Design review of the part built by this model. Coordinates are the model's own, in mm. Coordinates: 2 decimals unless noted, no trailing zeros. Loops run counter-clockwise (first coordinate to the right, second up) from the corner with the lowest first, then second, coordinate; pieces in that order, holes last. Notation, with made-up numbers: M 16.25,-12.75 L 53.25,-12.75 A10 ccw 53.25,-4.75 Z; hole C 20,37.25 d9. An arc over 180 degrees is marked long. Answer as CSV lines item,"result". Start each with the question number.
from build123d import *

# Parameters (mm, degrees)
SKETCH_1_R             = 175
EXTRUDE_1_DEPTH        = 3
CUT_EXTRUDE_1_DEPTH    = 3
FILLET_1_R             = 5
FILLET_2_R             = 5
FILLET_3_R             = 5
SKETCH_5_R             = 1.5
CUT_EXTRUDE_4_DEPTH    = 3
SKETCH_6_R             = 1.5
CUT_EXTRUDE_5_DEPTH    = 3
SKETCH_7_W             = 30
SKETCH_7_H             = 108
CUT_EXTRUDE_6_DEPTH    = 3
SKETCH_8_R             = 1.5
CUT_EXTRUDE_7_DEPTH    = 3
SKETCH_9_R             = 1.5
CUT_EXTRUDE_8_DEPTH    = 10
SKETCH_10_R            = 1.6
CUT_EXTRUDE_9_DEPTH    = 10
SKETCH_11_W            = 15
SKETCH_11_H            = 30
CUT_EXTRUDE_10_DEPTH   = 10
SKETCH_17_R            = 1.5
CUT_EXTRUDE_12_DEPTH   = 4
SKETCH_29_R            = 1.5
CUT_EXTRUDE_6879_DEPTH = 4
SKETCH_30_R            = 1.5
CUT_EXTRUDE_7056_DEPTH = 4
SKETCH_31_R            = 1.5
CUT_EXTRUDE_7256_DEPTH = 4
SKETCH_32_R            = 1.5
WEB_DEPTH              = 4


with BuildPart() as part:
    # ｽｹｯﾁ1 → ﾎﾞｽ - 押し出し1 (new body)
    with BuildSketch(Plane.XY):
        Circle(SKETCH_1_R)
    extrude(amount=EXTRUDE_1_DEPTH)

    # ｽｹｯﾁ2 → ｶｯﾄ - 押し出し1 (cut)
    with BuildSketch(Plane.XY.offset(3)):
        with BuildLine():
            Line((-60, 115), (0, 115))
            Line((0, 115), (0, 175))
            ThreePointArc((0, 175), (-30.465194158, 172.327803749), (-60, 164.392822228))
            Line((-60, 164.392822228), (-60, 115))
        make_face()
        with BuildLine():
            Line((0, 175), (0, 115))
            Line((0, 115), (60, 115))
            Line((60, 115), (60, 164.392822228))
            ThreePointArc((60, 164.392822228), (30.465194158, 172.327803749), (0, 175))
        make_face()
        with BuildLine():
            Line((0, -175), (0, -115))
            Line((0, -115), (-60, -115))
            Line((-60, -115), (-60, -164.392822228))
            ThreePointArc((-60, -164.392822228), (-30.465194158, -172.327803749), (0, -175))
        make_face()
        with BuildLine():
            Line((60, -115), (0, -115))
            Line((0, -115), (0, -175))
            ThreePointArc((0, -175), (30.465194158, -172.327803749), (60, -164.392822228))
            Line((60, -164.392822228), (60, -115))
        make_face()
    extrude(amount=-CUT_EXTRUDE_1_DEPTH, mode=Mode.SUBTRACT)

    # ﾌｨﾚｯﾄ1
    fillet_1_edges = [part.edges().sort_by_distance(p)[0] for p in [
        (-60, 164.392822228, 1.5),
    ]]
    fillet(fillet_1_edges, radius=FILLET_1_R)

    # ﾌｨﾚｯﾄ2
    fillet_2_edges = [part.edges().sort_by_distance(p)[0] for p in [
        (-60, 115, 1.5),
        (60, 164.392822228, 1.5),
        (60, 115, 1.5),
    ]]
    fillet(fillet_2_edges, radius=FILLET_2_R)

    # ﾌｨﾚｯﾄ3
    fillet_3_edges = [part.edges().sort_by_distance(p)[0] for p in [
        (-60, -115, 1.5),
        (60, -115, 1.5),
        (60, -164.392822228, 1.5),
        (-60, -164.392822228, 1.5),
    ]]
    fillet(fillet_3_edges, radius=FILLET_3_R)

    # ｽｹｯﾁ5 → ｶｯﾄ - 押し出し4 (cut)
    with BuildSketch(Plane.XY.offset(3)):
        with Locations((-100, -115)):
            Circle(SKETCH_5_R)
        with Locations((100, -115)):
            Circle(SKETCH_5_R)
        with Locations((100, 115)):
            Circle(SKETCH_5_R)
        with Locations((-100, 115)):
            Circle(SKETCH_5_R)
    extrude(amount=-CUT_EXTRUDE_4_DEPTH, mode=Mode.SUBTRACT)

    # ｽｹｯﾁ6 → ｶｯﾄ - 押し出し5 (cut)
    with BuildSketch(Plane.XY.offset(3)):
        with Locations((-60, 54)):
            Circle(SKETCH_6_R)
        with Locations((60, 54)):
            Circle(SKETCH_6_R)
        with Locations((-60, -54)):
            Circle(SKETCH_6_R)
        with Locations((60, -54)):
            Circle(SKETCH_6_R)
    extrude(amount=-CUT_EXTRUDE_5_DEPTH, mode=Mode.SUBTRACT)

    # ｽｹｯﾁ7 → ｶｯﾄ - 押し出し6 (cut)
    with BuildSketch(Plane.XY.offset(3)):
        with Locations((-85, 0)):
            Rectangle(SKETCH_7_W, SKETCH_7_H)
    extrude(amount=-CUT_EXTRUDE_6_DEPTH, mode=Mode.SUBTRACT)

    # ｽｹｯﾁ8 → ｶｯﾄ - 押し出し7 (cut)
    with BuildSketch(Plane.XY.offset(3)):
        with Locations((-115, -67)):
            Circle(SKETCH_8_R)
        with Locations((-116.822468618, 0)):
            Circle(SKETCH_8_R)
        with Locations((-115, 67)):
            Circle(SKETCH_8_R)
    extrude(amount=-CUT_EXTRUDE_7_DEPTH, mode=Mode.SUBTRACT)

    # ｽｹｯﾁ9 → ｶｯﾄ - 押し出し8 (cut)
    with BuildSketch(Plane.XY.offset(3)):
        with Locations((-65, 37)):
            Circle(SKETCH_9_R)
        with Locations((20, 41)):
            Circle(SKETCH_9_R)
        with Locations((-65, -38)):
            Circle(SKETCH_9_R)
        with Locations((20, -40)):
            Circle(SKETCH_9_R)
    extrude(amount=-CUT_EXTRUDE_8_DEPTH, mode=Mode.SUBTRACT)

    # ｽｹｯﾁ10 → ｶｯﾄ - 押し出し9 (cut)
    with BuildSketch(Plane.XY.offset(3)):
        with Locations((111.643659725, -125.921059639)):
            Circle(SKETCH_10_R)
        with Locations((122.679794489, -115.037952538)):
            Circle(SKETCH_10_R)
        with Locations((168, 7.75)):
            Circle(SKETCH_10_R)
        with Locations((168, -7.75)):
            Circle(SKETCH_10_R)
        with Locations((111.56768007, 125.844011632)):
            Circle(SKETCH_10_R)
        with Locations((122.679794489, 115.037952538)):
            Circle(SKETCH_10_R)
    extrude(amount=-CUT_EXTRUDE_9_DEPTH, mode=Mode.SUBTRACT)

    # ｽｹｯﾁ11 → ｶｯﾄ - 押し出し10 (cut)
    with BuildSketch(Plane.XY.offset(3)):
        with Locations((81.317279836, 81.317279836)):
            Rectangle(SKETCH_11_W, SKETCH_11_H)
        with Locations((81.317279836, -81.317279836)):
            Rectangle(SKETCH_11_W, SKETCH_11_H)
    extrude(amount=-CUT_EXTRUDE_10_DEPTH, mode=Mode.SUBTRACT)

    # ｽｹｯﾁ17 → ｶｯﾄ - 押し出し12 (cut, through all)
    with BuildSketch(Plane.XY.offset(3)):
        with Locations((-7.75, 90)):
            Circle(SKETCH_17_R)
        with Locations((7.75, 90)):
            Circle(SKETCH_17_R)
        with Locations((7.45, -90)):
            Circle(SKETCH_17_R)
        with Locations((-7.45, -90)):
            Circle(SKETCH_17_R)
    extrude(amount=-CUT_EXTRUDE_12_DEPTH, mode=Mode.SUBTRACT)

    # ｽｹｯﾁ29 → Cut-Extrude 6879 (cut, through all)
    with BuildSketch(Plane.XY.offset(3)):
        with Locations((80, 145)):
            Circle(SKETCH_29_R)
        with Locations((80, 129.5)):
            Circle(SKETCH_29_R)
    extrude(amount=-CUT_EXTRUDE_6879_DEPTH, mode=Mode.SUBTRACT)

    # ｽｹｯﾁ30 → Cut-Extrude 7056 (cut, through all)
    with BuildSketch(Plane.XY.offset(3)):
        with Locations((80, -129.5)):
            Circle(SKETCH_30_R)
        with Locations((80, -145)):
            Circle(SKETCH_30_R)
    extrude(amount=-CUT_EXTRUDE_7056_DEPTH, mode=Mode.SUBTRACT)

    # ｽｹｯﾁ31 → Cut-Extrude 7256 (cut, through all)
    with BuildSketch(Plane.XY.offset(3)):
        with Locations((-140, 37.5)):
            Circle(SKETCH_31_R)
        with Locations((-140, -37.5)):
            Circle(SKETCH_31_R)
    extrude(amount=-CUT_EXTRUDE_7256_DEPTH, mode=Mode.SUBTRACT)

    # ｽｹｯﾁ32 → WEBカメラ (cut, through all)
    with BuildSketch(Plane.XY.offset(3)):
        with Locations((150, 10)):
            Circle(SKETCH_32_R)
        with Locations((150, -10)):
            Circle(SKETCH_32_R)
    extrude(amount=-WEB_DEPTH, mode=Mode.SUBTRACT)


solid = part.part
Item 1: For pin 1 (1.5 mm diameter, centred on y = -37.5, z = 0.5, fed in from +X); pin 2 (0.9 mm diameter, centred on y = -144, z = 1, fed in from +X); pin 3 (1.5 mm diameter, centred on x = 47, z = 1, fed in from -Y), all flat-tipped, find the tip position at first contact; note any pin that passes through.
Item 2: Mouldability with a two-part tool opening along X and no side actions: class faces 1 (the face through (-174.976, 2.887, 1.479)), 2 (the face through (-2, 2, 0)), 3 (the face through (174.976, -2.887, 1.479)) as released by +X, released by -X, zero draft, split by the parting line, or undercut.
Item 3: Add section A-A (x = -147.5). Give the boundary of the cut face in (y, z).
Item 4: For line 1 along Y through (x, z) = (150, 1.75); line 2 along X through (y, z) = (129.5, 1.15); line 3 along Y through (x, z) = (40, 1.95), list the stretches that pass through material, from the lowest coordinate up. Write a range as from..to.
Item 5: Add section B-B (z = 2.1). Give the number of separate pieces and of enclosed holes in the cut face, plus the area to 3 significant figures.
Response:
1,pin 1,"x = 171.1"
1,pin 2,"x = 100.09"
1,pin 3,"y = -115"
2,face 1,"released by -X"
2,face 2,"zero draft"
2,face 3,"released by +X"
3,outline,"M -94.17,0 L 94.17,0 L 94.17,3 L -94.17,3 Z"
4,line 1,"-90.14..-11.5, -8.5..8.5, 11.5..90.14"
4,line 2,"-117.71..-60, 60..78.5, 81.5..117.71"
4,line 3,"-115..115"
5,separate pieces,"1"
5,enclosed holes,"36"
5,area,"78,200 mm²"
